Could you check a few things on this model? Use its own coordinates, in mm. Face numbers are marked on the shaded views. A direction names the side the tool comes from. Give positions to 0.01 mm unless a question says otherwise; leave off trailing zeros. Order: outer loops, then holes, each group sorted by start corner. A loop starts at its lowest first (then second) coordinate and runs counter-clockwise, first axis right, second up. Notation, with made-up numbers: (64.25, 5.25) -> (93.25, 5.25) arc R21 ccw to (93.25, 29.25) -> close; hole circle Ø11 at (-12.5, -3). An arc over 180 degrees is marked (long way). Answer as CSV lines item,"result". Start each with the question number.
(1) Will this pin go through, and if not, where does the flat tip stop? pin 1 Ø19 at (x, y) = (36.5, 30) entering from +Z.
(2) I want a section at B-B (y = 27.5). Please give me the cut outline in (x, z), plus the area to 3 significant figures.
(3) On a 3-axis mill with a long thin cutter (end or side, diameter ignored), from which of +Z, -Z, +X, -X, +Y, -Y can I reach the whole of each face in a straight line? I mean the marked faces 1 and 2. Say none if no direction works.
(4) I need wall thicknesses on L1, parallel to Y at x = 14, z = 14; L2, parallel to X at y = 48.5, z = 6; L3, parallel to X at y = 7, z = 7.5. Which ranges of each line are inside material? Lowest first, please.
(5) I want a section at A-A (x = 36.5). Please give me the cut outline in (y, z).
(6) We'd pull the mould along X, two halves only. Please class the marked faces 3, 4 and 5: released by +X, released by -X, zero draft, split by the parting line, or undercut.
```python
from build123d import *

# Parameters (mm, degrees)
F0_W      = 55
F0_H      = 55
F1_DEPTH  = 2
F2_W      = 0.8393637836
F2_H      = 13.1056420505
F2_W_2    = 14.2980124801
F2_H_2    = 1.318924129
F2_W_3    = 17.9352443665
F2_H_3    = 1.0551437736
F2_W_4    = 0.6528366357
F2_H_4    = 5.0601772964
F2_W_5    = 1.0258853436
F2_H_5    = 24.1364017129
F2_W_6    = 0.7460992783
F2_H_6    = 12.0504982769
F2_W_7    = 8.0205630511
F2_W_8    = 9.2725682259
F2_H_7    = 0.9232535958
F2_W_9    = 0.6528384984
F2_H_8    = 9.0530256927
F2_W_10   = 9.2923234403
F2_H_9    = 0.8714348078
F3_DEPTH  = 25
F5_DEPTH  = 2
F7_DEPTH  = 25
F8_W      = 57
F8_H      = 2
F9_DEPTH  = 2
F10_W     = 2
F10_H     = 57
F11_DEPTH = 25
F13_DEPTH = 2
F15_DEPTH = 25
F17_DEPTH = 2
F19_DEPTH = 25
F20_W     = 5.9659110848
F20_H     = 4.5738629997
F21_DEPTH = 25
F24_DEPTH = 2
F26_DEPTH = 2


with BuildPart() as f1:
    # F0 (on Top) → F1 (new body)
    with BuildSketch(Plane.XY):
        with Locations((27.5, 27.5)):
            Rectangle(F0_W, F0_H)
    extrude(amount=F1_DEPTH)

    # F2 (on face) → F3 (join)
    with BuildSketch(Plane.XY.offset(2)):
        with Locations((46.2403725833, 6.5528210253)):
            Rectangle(F2_W, F2_H)
        with Locations((7.1490062401, 45.6831902266)):
            Rectangle(F2_W_2, F2_H_2)
        Polygon((15.0441108271, 46.3426522911), (14.2980124801, 46.3426522911), (14.2980124801, 45.0237281621), (14.2980124801, 19.9640728533), (15.0441108271, 19.9640728533), align=None)
        Polygon((15.0441108271, 19.9640728533), (14.2980124801, 19.9640728533), (7.4898591265, 19.9640728533), (7.4898591265, 18.9089290798), (15.0441108271, 18.9089290798), align=None)
        Polygon((7.4898591265, 18.9089290798), (7.4898591265, 19.9640728533), (7.4898591265, 36.5825779736), (6.6504976712, 36.5825779736), (6.6504976712, 18.9089290798), align=None)
        with Locations((8.9676221833, 8.8850706816)):
            Rectangle(F2_W_3, F2_H_3)
        with Locations((9.9613117054, 2.5300886482)):
            Rectangle(F2_W_4, F2_H_4)
        Polygon((22.4118363112, 55), (21.5724762529, 55), (21.5724762529, 18.9089290798), (22.4118363112, 18.9089290798), (22.4118363112, 20.2278606594), align=None)
        Polygon((34.1628938913, 20.2278606594), (22.4118363112, 20.2278606594), (22.4118363112, 18.9089290798), (35.1887792349, 18.9089290798), (35.1887792349, 20.2278606594), align=None)
        with Locations((34.6758365631, 32.2960615158)):
            Rectangle(F2_W_5, F2_H_5)
        Polygon((28.5671520978, 44.3642623723), (34.1628938913, 44.3642623723), (35.1887792349, 44.3642623723), (35.1887792349, 45.5512963235), (28.5671520978, 45.5512963235), align=None)
        Polygon((28.5671520978, 30.6474007666), (28.5671520978, 44.3642623723), (28.5671520978, 45.5512963235), (27.5412686169, 45.5512963235), (27.5412686169, 30.6474007666), align=None)
        with Locations((30.0593515858, 6.0252491385)):
            Rectangle(F2_W_6, F2_H_6)
        with Locations((30.0593515858, 12.5780701637)):
            Rectangle(F2_W_6, F2_H_3)
        with Locations((34.4426827505, 12.5780701637)):
            Rectangle(F2_W_7, F2_H_3)
        Polygon((38.4529642761, 13.1056420505), (38.4529642761, 12.0504982769), (39.4788496196, 12.0504982769), (39.4788496196, 49.376193434), (38.4529642761, 49.376193434), align=None)
        with Locations((50.3637158871, 40.7372042537)):
            Rectangle(F2_W_8, F2_H_7)
        with Locations((48.1056179851, 50.4734871536)):
            Rectangle(F2_W_9, F2_H_8)
        with Locations((50.3538382798, 22.9402892292)):
            Rectangle(F2_W_10, F2_H_9)
    extrude(amount=F3_DEPTH)

    # F4 (on face) → F5 (join)
    with BuildSketch(Plane.XZ):
        Polygon((9.6348933876, 2), (0, 2), (0, 0), (55, 0), (55, 2), (46.6600544751, 2), (45.8206906915, 2), (30.432401225, 2), (29.6863019466, 2), (10.2877300233, 2), align=None)
    extrude(amount=F5_DEPTH)

    # F6 (on face) → F7 (join)
    with BuildSketch(Plane.XY.offset(2)):
        Polygon((9.6348933876, 0), (0, 0), (0, -2), (55, -2), (55, 0), (46.6600544751, 0), (45.8206906915, 0), (30.432401225, 0), (29.6863019466, 0), (10.2877300233, 0), align=None)
    extrude(amount=F7_DEPTH)

    # F8 (on face) → F9 (join)
    with BuildSketch(Plane(origin=(0, 0, 0), x_dir=(0, -1, 0), z_dir=(-1, 0, 0))):
        with Locations((-26.5, 1)):
            Rectangle(F8_W, F8_H)
    extrude(amount=F9_DEPTH)

    # F10 (on face) → F11 (join)
    with BuildSketch(Plane.XY.offset(2)):
        with Locations((-1, 26.5)):
            Rectangle(F10_W, F10_H)
    extrude(amount=F11_DEPTH)

    # F12 (on face) → F13 (join)
    with BuildSketch(Plane(origin=(0, 55, 0), x_dir=(-1, 0, 0), z_dir=(0, 1, 0))):
        Polygon((-55, 0), (2, 0), (2, 2), (0, 2), (-21.5724762529, 2), (-22.4118363112, 2), (-47.779198736, 2), (-48.4320372343, 2), (-55, 2), align=None)
    extrude(amount=F13_DEPTH)

    # F14 (on face) → F15 (join)
    with BuildSketch(Plane.XY.offset(2)):
        Polygon((55, 55), (55, 57), (-2, 57), (-2, 55), (0, 55), (21.5724762529, 55), (22.4118363112, 55), (47.779198736, 55), (48.4320372343, 55), align=None)
    extrude(amount=F15_DEPTH)

    # F16 (on face) → F17 (join)
    with BuildSketch(Plane.YZ.offset(55)):
        Polygon((-2, 2), (-2, 0), (57, 0), (57, 2), (55, 2), (41.1988310516, 2), (40.2755774558, 2), (23.376006633, 2), (22.5045718253, 2), (0, 2), align=None)
    extrude(amount=F17_DEPTH)

    # F18 (on face) → F19 (join)
    with BuildSketch(Plane.XY.offset(2)):
        Polygon((57, -2), (57, 57), (55, 57), (55, 55), (55, 41.1988310516), (55, 40.2755774558), (55, 23.376006633), (55, 22.5045718253), (55, 0), (55, -2), align=None)
    extrude(amount=F19_DEPTH)

    # F20 (on face) → F21 (cut)
    with BuildSketch(Plane.XY.offset(2)):
        with Locations((6.1647732509, 50.411934033)):
            Rectangle(F20_W, F20_H)
    extrude(amount=-F21_DEPTH, mode=Mode.SUBTRACT)

    # F23 (on face) → F24 (join, through all)
    with BuildSketch(Plane.YZ.offset(57)):
        with BuildLine():
            Line((22.5, 27), (32.5, 27))
            ThreePointArc((32.5, 27), (27.5, 32), (22.5, 27))
        make_face()
        with BuildLine():
            Line((57, 27), (32.5, 27))
            ThreePointArc((32.5, 27), (27.5, 22), (22.5, 27))
            Line((22.5, 27), (-2, 27))
            Line((-2, 27), (-2, 0))
            Line((-2, 0), (57, 0))
            Line((57, 0), (57, 27))
        make_face()
    extrude(amount=-F24_DEPTH)

    # F25 (on face) → F26 (join, through all)
    with BuildSketch(Plane.YZ):
        with BuildLine():
            Line((22.2181853652, 27), (32.2181853652, 27))
            ThreePointArc((32.2181853652, 27), (27.2181853652, 32), (22.2181853652, 27))
        make_face()
    extrude(amount=-F26_DEPTH)


solid = f1.part
```
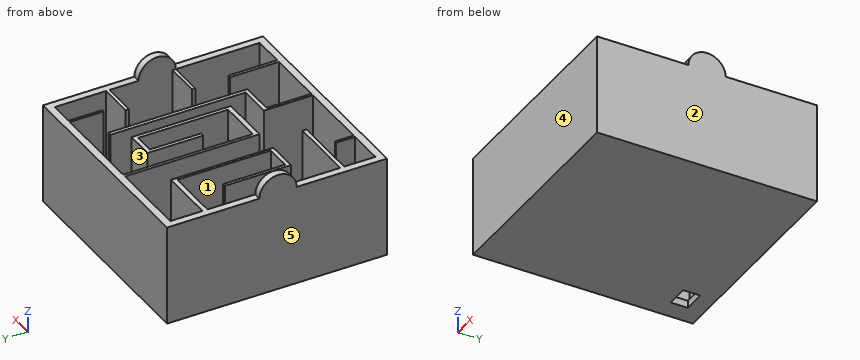
Final values:
1,pin 1,"z = 27"
2,outline,"(-2, 0) -> (57, 0) -> (57, 32) -> (55, 32) -> (55, 2) -> (39.48, 2) -> (39.48, 27) -> (38.45, 27) -> (38.45, 2) -> (35.19, 2) -> (35.19, 27) -> (34.16, 27) -> (34.16, 2) -> (22.41, 2) -> (22.41, 27) -> (21.57, 27) -> (21.57, 2) -> (15.04, 2) -> (15.04, 27) -> (14.3, 27) -> (14.3, 2) -> (7.49, 2) -> (7.49, 27) -> (6.65, 27) -> (6.65, 2) -> (0, 2) -> (0, 31.99) -> (-2, 31.99) -> close"
2,area,"350 mm²"
3,face 1,"+Z"
3,face 2,"+Z, -Z, +X, +Y, -Y"
4,L1,"-2 to 0, 8.36 to 9.41, 18.91 to 19.96, 45.02 to 46.34, 55 to 57"
4,L2,"-2 to 0, 21.57 to 22.41, 38.45 to 39.48, 47.78 to 48.43, 55 to 57"
4,L3,"-2 to 0, 29.69 to 30.43, 45.82 to 46.66, 55 to 57"
5,outline,"(-2, 0) -> (57, 0) -> (57, 27) -> (55, 27) -> (55, 2) -> (13.11, 2) -> (13.11, 27) -> (12.05, 27) -> (12.05, 2) -> (0, 2) -> (0, 27) -> (-2, 27) -> close"
6,face 3,"undercut"
6,face 4,"zero draft"
6,face 5,"released by -X"
